Input: part model. Units: mm. Frame: model coordinates. Give positions to 0.01 mm unless a question says otherwise; leave off trailing zeros. Loops run counter-clockwise (first coordinate to the right, second up) from the corner with the lowest first, then second, coordinate; pieces in that order, holes last. Notation, with made-up numbers: M 58,-30 L 100,-30 A14 ccw 100,-5 Z; hole C 33.25,-5 d10. An arc over 180 degrees is marked long. Return JSON: item names as keys, results as strings. Group by question number.
Autodesk Inventor part; units mm, degrees
ref_plane "YZ Plane" through (0, 0, 0) normal (1, 0, 0) x (0, 1, 0)
ref_plane "XZ Plane" through (0, 0, 0) normal (0, 1, 0) x (-1, 0, 0)
ref_plane "XY Plane" through (0, 0, 0) normal (0, 0, 1) x (1, 0, 0)
sketch "Sketch1" plane through (0, 0, 0) normal (0, 0, 1) x (1, 0, 0)
  line L0 (-1.75, 0) -> (1.75, 0) construction
  line L1 (-1.75, -1) -> (1.75, -1)
  line L2 (1.75, 1) -> (-1.75, 1)
  arc A0 (-1.75, 1) -> (-1.75, -1) centre (-1.75, 0) ccw
  arc A1 (1.75, -1) -> (1.75, 1) centre (1.75, 0) ccw
  circle A2 centre (0, 0) radius 0.875
  circle A3 centre (1.75, 0) radius 0.875
  circle A4 centre (-1.75, 0) radius 0.875
  point P0 (-0.875, 0)
  point P1 (0.875, 0)
  dimension "d0" = 1.75
  dimension "d1" = 2
  dimension "d4" = 1.75
  dimension "d5" = 1.75
  dimension "d6" = 1.75
extrude "Extrusion1" add sketch "Sketch1" along normal blind 16.75 contours A0 L2 A1 L1 | A2 | A4 | A3
extrude "Extrusion2" add sketch "Sketch1" against normal blind 10 contours A2 | A4 | A3
properties part number "Cable Sleeve" material "Rubber, Silicone"
Item 1: First-contact query: pin 1 Ø1.5 at (x, z) = (-2, -2) entering from +Y (3 decimals); pin 2 Ø1 at (x, z) = (1.5, -6) entering from -Y (3 decimals). Flat tips, straight axial feed; report the tip coordinate or a pass-through.
Item 2: Section D-D, the plane x = 2. Return loops of the section in (y, z).
Item 3: Section C-C, the plane z = 6. Return loops of the section in (x, y).
Item 4: Pull-direction query (X, two-part tool) for faces 1 (the face through (2.75, 0.02, 8.26)), 2 (the face through (0, 1, 8)), 3 (the face through (-0.019, -0.875, -4.93)), 4 (the face through (-2.75, -0.02, 8.26)); classes: pulls with the +X half, pulls with the -X half, needs draft (parallel to the pull), parting line crosses it, or undercut.
Item 5: Section A-A, the plane x = 0. Return loops of the section in (y, z) (3 decimals), then the cut area to 3 significant figures.
Item 6: Material intervals for line 1 (X direction, y = 0.6, z = -4); line 2 (X direction, y = 0.55, z = -4.5); line 3 (Y direction, x = 1, z = -6.75), sorted ascending. Write a range as from..to.
Answer below:
{
 "1": {"pin 1": "y = 0.875", "pin 2": "y = -0.875"},
 "2": {"outline": "M -0.97,0 L -0.84,0 L -0.84,-10 L 0.84,-10 L 0.84,0 L 0.97,0 L 0.97,16.75 L -0.97,16.75 Z"},
 "3": {"outline": "M -1.75,-1 L 1.75,-1 A1 ccw 1.75,1 L -1.75,1 A1 ccw Z"},
 "4": {"face 1": "pulls with the +X half", "face 2": "needs draft", "face 3": "undercut", "face 4": "pulls with the -X half"},
 "5": {"outline": "M -1,0 L -0.875,0 L -0.875,-10 L 0.875,-10 L 0.875,0 L 1,0 L 1,16.75 L -1,16.75 Z", "area": "51.0 mm^2"},
 "6": {"line 1": "-2.39..-1.11, -0.64..0.64, 1.11..2.39", "line 2": "-2.43..-1.07, -0.68..0.68, 1.07..2.43", "line 3": "-0.45..0.45"}
}
